```python
from build123d import *

# Parameters (mm, degrees)
SKETCH1_R           = 25.7175
SKETCH1_R_2         = 20.6375
BOSS_EXTRUDE1_DEPTH = 8.89
BOSS_EXTRUDE2_START = 3.175
SKETCH2_R           = 25.7175
SKETCH2_R_2         = 12.7
BOSS_EXTRUDE2_DEPTH = 3.175
BOSS_EXTRUDE3_START = -3.175
SKETCH3_R           = 3.175
BOSS_EXTRUDE3_DEPTH = 3.175


with BuildPart() as part:
    # Sketch1 → Boss-Extrude1 (new body)
    with BuildSketch(Plane(origin=(0, 0, 0), x_dir=(1, 0, 0), z_dir=(0, 1, 0))):
        with Locations(Location((0, 0, 0), (0, 0, 270))):
            Circle(SKETCH1_R)
        with Locations(Location((0, 0, 0), (0, 0, 270))):
            Circle(SKETCH1_R_2, mode=Mode.SUBTRACT)
    extrude(amount=BOSS_EXTRUDE1_DEPTH)

    # Sketch2 → Boss-Extrude2 (add)
    with BuildSketch(Plane.XZ.offset(BOSS_EXTRUDE2_START)):
        with Locations(Location((0, 0, 0), (0, 0, 270))):
            Circle(SKETCH2_R)
        with Locations(Location((0, 0, 0), (0, 0, 270))):
            Circle(SKETCH2_R_2, mode=Mode.SUBTRACT)
    extrude(amount=-BOSS_EXTRUDE2_DEPTH)

    # Sketch3 → Boss-Extrude3 (add)
    # profile 1 of 2: a face of its own
    with BuildSketch(Plane(origin=(0, 8.89, 0), x_dir=(1, 0, 0), z_dir=(0, 1, 0)).offset(BOSS_EXTRUDE3_START)):
        with BuildLine():
            Line((22.362911399, 12.7), (41.123499094, 9.392002215))
            ThreePointArc((41.123499094, 9.392002215), (49.004324689, 0), (41.123499094, -9.392002215))
            Line((41.123499094, -9.392002215), (22.362911399, -12.7))
            ThreePointArc((22.362911399, -12.7), (25.7175, 0), (22.362911399, 12.7))
        make_face()
        with Locations(Location((39.467435701, 0, 0), (0, 0, 270))):
            Circle(SKETCH3_R, mode=Mode.SUBTRACT)
    # profile 2 of 2: a face of its own
    with BuildSketch(Plane(origin=(0, 8.89, 0), x_dir=(1, 0, 0), z_dir=(0, 1, 0)).offset(BOSS_EXTRUDE3_START)):
        with BuildLine():
            Line((-22.362911399, -12.7), (-41.123499094, -9.392002215))
            ThreePointArc((-41.123499094, -9.392002215), (-49.004324689, 0), (-41.123499094, 9.392002215))
            Line((-41.123499094, 9.392002215), (-22.362911399, 12.7))
            ThreePointArc((-22.362911399, 12.7), (-25.7175, 0), (-22.362911399, -12.7))
        make_face()
        with Locations(Location((-39.467435701, 0, 0), (0, 0, 90))):
            Circle(SKETCH3_R, mode=Mode.SUBTRACT)
    extrude(amount=BOSS_EXTRUDE3_DEPTH)


solid = part.part
```
For this review, take the finished solid that the model builds, in its own axes (mm). A direction names the side the tool comes from. Coordinates: 2 decimals unless noted, no trailing zeros. Write each loop counter-clockwise with the first axis right and the second up, starting at its lowest first coordinate (ties: lowest second). Pieces come first, ordered by that corner, then holes. Notation, with made-up numbers: (39.5, 72.5) - (54.5, 72.5) arc R12 cw to (54.5, 84.5) - close; hole circle Ø2 at (-14, 21.25). An arc over 180 degrees is marked (long way). Put each result on its own line as item: value.
1. Wall thickness on probe 1 along X at (y, z) = (-1, 0); probe 2 along Y at (x, z) = (43, 2) (3 decimals); probe 3 along Z at (x, y) = (8, 6.5): over which ranges is each line inside the solid? List them lowest first.
Values found:
probe 1: -25.72 to -12.7, 12.7 to 25.72
probe 2: 5.715 to 8.89
probe 3: -24.44 to -19.02, 19.02 to 24.44
2. Add section D-D, the plane y = -1.25. Give the boundary of the cut face in (x, z) (1 decimal).
Values found:
outline: circle Ø51.4 at (0, 0); hole circle Ø25.4 at (0, 0)
3. For pin 1 (5 mm diameter, centred on x = 28.5, y = 7.5, fed in from +Z); pin 2 (7.5 mm diameter, centred on x = 35, z = 0.5, fed in from -Y) (3 decimals); pin 3 (1.5 mm diameter, centred on y = -1, z = -1, fed in from +X), all flat-tipped, find the tip position at first contact; note any pin that passes through.
Values found:
pin 1: z = 12.06
pin 2: y = 5.715
pin 3: x = 25.72
4. Add section C-C, the plane z = 6.5. Give the boundary of the cut face in (x, y) (3 decimals).
Values found:
outline: (-46.446, 5.715) - (-24.883, 5.715) - (-24.883, -3.175) - (-10.911, -3.175) - (-10.911, 0) - (-19.587, 0) - (-19.587, 8.89) - (-46.446, 8.89) - close; (10.911, -3.175) - (24.883, -3.175) - (24.883, 5.715) - (46.446, 5.715) - (46.446, 8.89) - (19.587, 8.89) - (19.587, 0) - (10.911, 0) - close
5. Add section B-B, the plane z = 0. Give the boundary of the cut face in (x, y) (1 decimal).
Values found:
outline: (-49, 5.7) - (-42.6, 5.7) - (-42.6, 8.9) - (-49, 8.9) - close; (-36.3, 5.7) - (-25.7, 5.7) - (-25.7, -3.2) - (-12.7, -3.2) - (-12.7, 0) - (-20.6, 0) - (-20.6, 8.9) - (-36.3, 8.9) - close; (12.7, -3.2) - (25.7, -3.2) - (25.7, 5.7) - (36.3, 5.7) - (36.3, 8.9) - (20.6, 8.9) - (20.6, 0) - (12.7, 0) - close; (42.6, 5.7) - (49, 5.7) - (49, 8.9) - (42.6, 8.9) - close
6. Add section A-A, the plane x = 0. Give the boundary of the cut face in (y, z) (1 decimal), then the cut area to 3 significant figures.
Values found:
outline: (-3.2, -25.7) - (8.9, -25.7) - (8.9, -20.6) - (0, -20.6) - (0, -12.7) - (-3.2, -12.7) - close; (-3.2, 12.7) - (0, 12.7) - (0, 20.6) - (8.9, 20.6) - (8.9, 25.7) - (-3.2, 25.7) - close
area: 173 mm²
7. Mouldability with a two-part tool opening along X and no side actions: class faces 3 (the flat face through (32, 7, -11)), 4 (the cylindrical face through (-49.003, 7.28, 0.186)), 5 (the flat face through (36, 5.715, 0)), 6 (the cylindrical face through (-7.7, -1.6, 10.1)) as released by +X, released by -X, zero draft, split by the parting line, or undercut.
Values found:
face 3: released by +X
face 4: released by -X
face 5: zero draft
face 6: undercut
8. Machinability: for faces 1 (the cylindrical face through (-36.37, 7.28, 0.69)), 2 (the cylindrical face through (20.46, 4.38, -2.69)), which of the approach directions +Z, -Z, +X, -X, +Y, -Y give a long, thin tool a straight path to every point of the face, cutting with its end or side? Answer none if there is none.
Values found:
face 1: +Y, -Y
face 2: +Y
